```python
from build123d import *

# Parameters (mm, degrees)
BOSS_EXTRUDE2_DEPTH = 6.35
SKETCH3_R           = 3.3
SKETCH3_R_2         = 4
SKETCH3_R_3         = 61.9125
SKETCH3_R_4         = 18.75
CUT_EXTRUDE1_DEPTH  = 704.212713409


with BuildPart() as part:
    # Sketch2 → Boss-Extrude2 (new body)
    with BuildSketch(Plane(origin=(0, 0, 0), x_dir=(1, 0, 0), z_dir=(0, 1, 0))):
        Polygon((-672.391731841, 17.123030998), (-672.391731841, -205.808543922), (-220.848796652, -173.149778169), (-220.848796652, 17.123030998), align=None)
    extrude(amount=BOSS_EXTRUDE2_DEPTH)

    # Sketch3 → Cut-Extrude1 (cut, through all)
    with BuildSketch(Plane(origin=(0, 6.35, 0), x_dir=(1, 0, 0), z_dir=(0, 1, 0))):
        with Locations(Location((-403.939830292, -23.331851988, 0), (0, 0, 270))):
            Circle(SKETCH3_R)
        with Locations(Location((-625.491718045, -18.795833368, 0), (0, 0, 270))):
            Circle(SKETCH3_R)
        with Locations(Location((-359.363535158, -87.997654624, 0), (0, 0, 270))):
            Circle(SKETCH3_R_2)
        with Locations(Location((-384.432251936, -97.121921342, 0), (0, 0, 270))):
            Circle(SKETCH3_R_2)
        with Locations(Location((-334.294818381, -97.121921342, 0), (0, 0, 270))):
            Circle(SKETCH3_R_2)
        with Locations(Location((-537.163535159, -115.999131996, 0), (0, 0, 270))):
            Circle(SKETCH3_R_3)
        with Locations(Location((-359.363535158, -126.997654624, 0), (0, 0, 270))):
            Circle(SKETCH3_R_4)
    extrude(amount=-CUT_EXTRUDE1_DEPTH, mode=Mode.SUBTRACT)


solid = part.part
```
Check sheet for the modelled part. Datum: model origin and axes. Units: mm. Round coordinates to 2 decimals unless told otherwise and drop trailing zeros. Order: outer loops, then holes, each group sorted by start corner. A loop starts at its lowest first (then second) coordinate and runs counter-clockwise, first axis right, second up. Notation, with made-up numbers: (-12.5, 50.5) -> (29.5, 50.5) arc R18 ccw to (29.5, 78.5) -> close; hole circle Ø6 at (72, -33.75). An arc over 180 degrees is marked (long way). One line per item, written item: value. Start each with the question number.
Q1. Gauge pin test, flat end, axial feed: pin 1 Ø6 at (x, z) = (-625.49, 18.8) entering from -Y. Record the tip position at first contact, or that the pin passes through.
Q2. Cross-section at A-A (z = 58.5). Record the boundary of the cut face in (x, y), and give its area (3 significant figures).
Q3. Cross-section at B-B (x = -508.5). Record the boundary of the cut face in (y, z), and give its area (3 significant figures).
Q4. Cross-section at D-D (z = 130.5). Record the boundary of the cut face in (x, y), and give its area (3 significant figures).
Q5. Thickness scan on line 1 (X direction, y = 2.25, z = 139) (3 decimals); line 2 (Z direction, x = -406, y = 3.25); line 3 (Z direction, x = -531, y = 5.25). Record the ranges inside material, lowest first.
Q6. Cross-section at C-C (y = 4.5). Give the number of separate pieces and of enclosed holes in the cut face, and give its area (3 significant figures).
Q7. Mould release check, pull along X, two halves, no side actions. Record for faces 1 (the face through (-450, 0, 93)), 2 (the face through (-380.466, 3.219, 96.601)), 3 (the face through (-449.781, 3.131, 189.708)): pulls with the +X half, pulls with the -X half, needs draft (parallel to the pull), parting line crosses it, or undercut.
Completed:
1. pin 1: passes through
2. outline: (-672.39, 0) -> (-560.12, 0) -> (-560.12, 6.35) -> (-672.39, 6.35) -> close; (-514.21, 0) -> (-220.85, 0) -> (-220.85, 6.35) -> (-514.21, 6.35) -> close
2. area: 2,580 mm²
3. outline: (0, -17.12) -> (6.35, -17.12) -> (6.35, 61.12) -> (0, 61.12) -> close; (0, 170.88) -> (6.35, 170.88) -> (6.35, 193.95) -> (0, 193.95) -> close
3. area: 643 mm²
4. outline: (-672.39, 0) -> (-597.35, 0) -> (-597.35, 6.35) -> (-672.39, 6.35) -> close; (-476.97, 0) -> (-377.78, 0) -> (-377.78, 6.35) -> (-476.97, 6.35) -> close; (-340.94, 0) -> (-220.85, 0) -> (-220.85, 6.35) -> (-340.94, 6.35) -> close
4. area: 1,870 mm²
5. line 1: x = -672.392 to -594.645, -479.682 to -373.769, -344.958 to -220.849
5. line 2: z = -17.12 to 20.75, 25.91 to 186.54
5. line 3: z = -17.12 to 54.39, 177.6 to 195.58
6. separate pieces: 1
6. enclosed holes: 7
6. area: 79,900 mm²
7. face 1: needs draft
7. face 2: undercut
7. face 3: pulls with the +X half
